Can you work these out from the model? Positions are in its coordinate system, mm. A direction names the side the tool comes from. Coordinates: 2 decimals unless noted, no trailing zeros. Order: outer loops, then holes, each group sorted by start corner. A loop starts at its lowest first (then second) coordinate and runs counter-clockwise, first axis right, second up. Notation, with made-up numbers: (17, 47) - (26, 47) arc R10 ccw to (26, 55) - close; hole circle Ø9 at (27, 82). An arc over 180 degrees is marked (long way). Return JSON: item names as keys, results as strings. Group by question number.
1) For pin 1 Ø2 at (x, y) = (-3, 3.5) entering from +Z; pin 2 Ø5 at (x, z) = (-0.5, -70) entering from +Y; pin 3 Ø3 at (x, y) = (3.5, 3) entering from -Z, each with a flat end and sliding along its axis, tell me the tip position at first contact or that it passes through.
2) Imagine slicing it at C-C (z = -37). Write out the boundary of the cut face in (x, y).
3) Imagine slicing it at B-B (y = 4.85). Write out the boundary of the cut face in (x, z) (3 decimals).
4) Which directions (+Z, -Z, +X, -X, +Y, -Y) give clear straight access to the entire face, cutting with the end or side of a thin tool? Please do faces 4 (the face through (0.345, 1.479, 1.097)), 5 (the face through (-1.08, 3.62, 4.88)).
5) If we mould it in two halves opening along X, with no side actions, what happens to faces 1 (the face through (0, 1, -95)), 2 (the face through (-1, 3, 1)), 3 (the face through (2, 6, 2))? For each: pulls with the +X half, pulls with the -X half, needs draft (parallel to the pull), parting line crosses it, or undercut.
6) Imagine slicing it at A-A (x = 0). Write out the boundary of the cut face in (y, z) (3 decimals), and give its area (3 significant figures).
7) If I drill on line 1 along Z through (x, y) = (0.25, 4.25); line 2 along Y through (x, z) = (1.25, -39.5); line 3 along Z through (x, y) = (0.75, 0.45), over which ranges is the centre line in solid material (lowest first)?
```python
from build123d import *

# Parameters (mm, degrees)
CROQUIS1_R              = 1.15
SALIENTE_EXTRUIR1_DEPTH = 3
CROQUIS2_R              = 5
CROQUIS2_R_2            = 2.625
SALIENTE_EXTRUIR2_DEPTH = 3


with BuildPart() as part:
    # Croquis1 → Saliente-Extruir1 (new body)
    with BuildSketch(Plane(origin=(0, 0, 0), x_dir=(1, 0, 0), z_dir=(0, 1, 0))):
        with BuildLine():
            Line((-5, 0), (-5, 90))
            ThreePointArc((-5, 90), (0, 95), (5, 90))
            Line((5, 90), (5, 0))
            ThreePointArc((5, 0), (0, -5), (-5, 0))
        make_face()
        with Locations(Location((0, 0, 0), (0, 0, 270))):
            Circle(CROQUIS1_R, mode=Mode.SUBTRACT)
    extrude(amount=SALIENTE_EXTRUIR1_DEPTH)

    # Croquis2 → Saliente-Extruir2 (add)
    with BuildSketch(Plane(origin=(0, 3, 0), x_dir=(1, 0, 0), z_dir=(0, 1, 0))):
        Circle(CROQUIS2_R)
        with Locations(Location((0, 0, 0), (0, 0, 270))):
            Circle(CROQUIS2_R_2, mode=Mode.SUBTRACT)
    extrude(amount=SALIENTE_EXTRUIR2_DEPTH)


solid = part.part
```
Calculated:
{
 "1": {"pin 1": "z = 4.58", "pin 2": "y = 3", "pin 3": "z = -94.58"},
 "2": {"outline": "(-5, 0) - (5, 0) - (5, 3) - (-5, 3) - close"},
 "3": {"outline": "circle Ø10 at (0, 0); hole circle Ø5.25 at (0, 0)"},
 "4": {"face 4": "+Y, -Y", "face 5": "+Y"},
 "5": {"face 1": "parting line crosses it", "face 2": "undercut", "face 3": "needs draft"},
 "6": {"outline": "(0, -95) - (3, -95) - (3, -5) - (6, -5) - (6, -2.625) - (3, -2.625) - (3, -1.15) - (0, -1.15) - close; (0, 1.15) - (3, 1.15) - (3, 2.625) - (6, 2.625) - (6, 5) - (0, 5) - close", "area": "307 mm2"},
 "7": {"line 1": "-4.99 to -2.61, 2.61 to 4.99", "line 2": "0 to 3", "line 3": "-94.94 to -0.87, 0.87 to 4.94"}
}
